Geometry: final body of the model. Coordinates: model frame, mm. A direction names the side the tool comes from. Coordinates: 2 decimals unless noted, no trailing zeros. Order: outer loops, then holes, each group sorted by start corner. A loop starts at its lowest first (then second) coordinate and runs counter-clockwise, first axis right, second up. Notation, with made-up numbers: M 85.25,25 L 138.25,25 A18 ccw 138.25,46 Z; hole C 19.5,20 d2. An arc over 180 degrees is marked long. Use CSV: the item, a comma, the result in double quotes. Start each with the question number.
1. Pull-direction query (Y, two-part tool) for faces 1 (the cylindrical face through (-0.915, -0.899, -3.451)), 2 (the flat face through (1, 1.8, -3)), 3 (the flat face through (-1.2, 2, -4)); classes: pulls with the +Y half, pulls with the -Y half, needs draft (parallel to the pull), parting line crosses it, or undercut.
2. Section query B-B on x = 4. Return the cut outline in (y, z), and give its area (3 significant figures).
3. Material intervals for line 1 (X direction, y = 4, z = -6); line 2 (Y direction, x = 1.25, z = -0.5); line 3 (X direction, y = -0.25, z = -2), sorted ascending.
4. Section query C-C on y = 3.5. Return the cut outline in (x, z), and give its area (3 significant figures).
5. Section query A-A on z = -4. State how many separate pieces and enclosed holes the cut face has, and give its area (3 significant figures).
6. Section query D-D on z = 0.5. Return the cut outline in (x, y), and give its area (3 significant figures).
7. Set-up query: faces 4 (the flat face through (4, 2, 1)), 5 (the flat face through (1, 4, 0)). Return all of +Z, -Z, +X, -X, +Y, -Y with unobstructed straight access to the full face (end or side cutting, diameter ignored); none if empty.
from build123d import *

# Parameters (mm, degrees)
F0_W     = 2.4
F0_H     = 2.4
F0_W_2   = 1.2
F0_H_2   = 1.2
F1_DEPTH = 7
F2_DEPTH = 1
F3_R     = 1


# Not quite as in the source:
# - a feature names something its author has since deleted; it is built from what else it names


with BuildPart() as f1:
    # F0 (on Top) → F1 (new body)
    with BuildSketch(Plane.XY):
        Polygon((-1.2, 6), (-1.2, 2.4), (-1.2, -1.2), (2.4, -1.2), (4.8, -1.2), (8.4, -1.2), (8.4, 2.4), (8.4, 6), (4.8, 6), (2.4, 6), align=None)
        Polygon((2.4, 0), (0, 0), (0, 2.4), (0, 4.8), (2.4, 4.8), (4.8, 4.8), (7.2, 4.8), (7.2, 2.4), (7.2, 0), (4.8, 0), align=None, mode=Mode.SUBTRACT)
        with Locations((1.2, 3.6)):
            Rectangle(F0_W, F0_H)
        with Locations((1.2, 3.6)):
            Rectangle(F0_W_2, F0_H_2, mode=Mode.SUBTRACT)
        with Locations((3.6, 3.6)):
            Rectangle(F0_W, F0_H)
        with Locations((3.6, 3.6)):
            Rectangle(F0_W_2, F0_H_2, mode=Mode.SUBTRACT)
        with Locations((6, 3.6)):
            Rectangle(F0_W, F0_H)
        with Locations((6, 3.6)):
            Rectangle(F0_W_2, F0_H_2, mode=Mode.SUBTRACT)
        with Locations((6, 1.2)):
            Rectangle(F0_W, F0_H)
        with Locations((6, 1.2)):
            Rectangle(F0_W_2, F0_H_2, mode=Mode.SUBTRACT)
        with Locations((3.6, 1.2)):
            Rectangle(F0_W, F0_H)
        with Locations((3.6, 1.2)):
            Rectangle(F0_W_2, F0_H_2, mode=Mode.SUBTRACT)
        with Locations((1.2, 1.2)):
            Rectangle(F0_W, F0_H)
        with Locations((1.2, 1.2)):
            Rectangle(F0_W_2, F0_H_2, mode=Mode.SUBTRACT)
    extrude(amount=-F1_DEPTH)

    # F0 (on Top) → F2 (join)
    with BuildSketch(Plane.XY):
        Polygon((-1.2, 6), (-1.2, 2.4), (-1.2, -1.2), (2.4, -1.2), (4.8, -1.2), (8.4, -1.2), (8.4, 2.4), (8.4, 6), (4.8, 6), (2.4, 6), align=None)
        Polygon((2.4, 0), (0, 0), (0, 2.4), (0, 4.8), (2.4, 4.8), (4.8, 4.8), (7.2, 4.8), (7.2, 2.4), (7.2, 0), (4.8, 0), align=None, mode=Mode.SUBTRACT)
        with Locations((3.6, 3.6)):
            Rectangle(F0_W, F0_H)
        with Locations((3.6, 3.6)):
            Rectangle(F0_W_2, F0_H_2, mode=Mode.SUBTRACT)
        with Locations((6, 3.6)):
            Rectangle(F0_W, F0_H)
        with Locations((6, 3.6)):
            Rectangle(F0_W_2, F0_H_2, mode=Mode.SUBTRACT)
        with Locations((1.2, 3.6)):
            Rectangle(F0_W, F0_H)
        with Locations((1.2, 3.6)):
            Rectangle(F0_W_2, F0_H_2, mode=Mode.SUBTRACT)
        with Locations((1.2, 1.2)):
            Rectangle(F0_W, F0_H)
        with Locations((1.2, 1.2)):
            Rectangle(F0_W_2, F0_H_2, mode=Mode.SUBTRACT)
        with Locations((3.6, 1.2)):
            Rectangle(F0_W, F0_H)
        with Locations((3.6, 1.2)):
            Rectangle(F0_W_2, F0_H_2, mode=Mode.SUBTRACT)
        with Locations((6, 1.2)):
            Rectangle(F0_W, F0_H)
        with Locations((6, 1.2)):
            Rectangle(F0_W_2, F0_H_2, mode=Mode.SUBTRACT)
        with Locations((6, 3.6)):
            Rectangle(F0_W_2, F0_H_2)
        with Locations((3.6, 3.6)):
            Rectangle(F0_W_2, F0_H_2)
        with Locations((1.2, 3.6)):
            Rectangle(F0_W_2, F0_H_2)
        with Locations((1.2, 1.2)):
            Rectangle(F0_W_2, F0_H_2)
        with Locations((3.6, 1.2)):
            Rectangle(F0_W_2, F0_H_2)
        with Locations((6, 1.2)):
            Rectangle(F0_W_2, F0_H_2)
    extrude(amount=F2_DEPTH)

    # F3
    f3_edges = [f1.edges().sort_by_distance(p)[0] for p in [
        (-1.2, -1.2, -3),
        (-1.2, 2.4, 1),
        (3.6, -1.2, 1),
        (8.4, -1.2, -3),
        (8.4, 2.4, 1),
        (3.6, 6, 1),
        (8.4, 6, -3),
        (-1.2, 6, -3),
    ]]
    fillet(f3_edges, radius=F3_R)


solid = f1.part
Results list:
1,face 1,"pulls with the -Y half"
1,face 2,"undercut"
1,face 3,"needs draft"
2,outline,"M -1.2,-7 L 0.6,-7 L 0.6,0 L 1.8,0 L 1.8,-7 L 3,-7 L 3,0 L 4.2,0 L 4.2,-7 L 6,-7 L 6,0 A1 ccw 5,1 L -0.2,1 A1 ccw -1.2,0 Z"
2,area,"40.4 mm²"
3,line 1,"x = -1.2 to 0.6, 1.8 to 3, 4.2 to 5.4, 6.6 to 8.4"
3,line 2,"y = -1.2 to 0.6, 1.8 to 3, 4.2 to 6"
3,line 3,"x = -1.2 to 8.4"
4,outline,"M -1.2,-7 L 0.6,-7 L 0.6,0 L 1.8,0 L 1.8,-7 L 3,-7 L 3,0 L 4.2,0 L 4.2,-7 L 5.4,-7 L 5.4,0 L 6.6,0 L 6.6,-7 L 8.4,-7 L 8.4,0 A1 ccw 7.4,1 L -0.2,1 A1 ccw -1.2,0 Z"
4,area,"51.2 mm²"
5,separate pieces,"1"
5,enclosed holes,"6"
5,area,"59.6 mm²"
6,outline,"M -1.07,-0.2 A0.87 ccw -0.2,-1.07 L 7.4,-1.07 A0.87 ccw 8.27,-0.2 L 8.27,5 A0.87 ccw 7.4,5.87 L -0.2,5.87 A0.87 ccw -1.07,5 Z"
6,area,"64.0 mm²"
7,face 4,"+Z, +X, -X, +Y, -Y"
7,face 5,"-Z"
